Source: CAD feature listing. Evaluate the final solid. Frame: model axes, mm. Coordinates: 2 decimals unless noted, no trailing zeros. Loops run counter-clockwise (first coordinate to the right, second up) from the corner with the lowest first, then second, coordinate; pieces in that order, holes last. Notation, with made-up numbers: M -12,16 L 35,16 A12 cw 35,28 Z; hole C -17.75,87 d9. An arc over 180 degrees is marked long. One line per question, with ' | ' between items. Start each with the question number.
1. Section query C-C, the plane x = -10. Output: boundary loops of the cut face in (y, z), and give its area (3 significant figures).
2. Section query A-A, the plane z = -2.5. Output: boundary loops of the cut face in (x, y).
3. Ray query, probe 1 along X at (y, z) = (-2, -7.5); probe 2 along Z at (x, y) = (-10.75, -2.3); probe 3 along X at (y, z) = (-2.1, -5.25). Return the intervals inside material, ascending.
4. Section query B-B, the plane y = -1.2. Output: boundary loops of the cut face in (x, z), and give its area (3 significant figures).
5. Pin query (flat end, axial travel): P1, Ø8, axis at x = 2, z = -15, coming from the +Y side. Return the tip coordinate at first contact, or that it passes through.
```python
from build123d import *

# Parameters (mm, degrees)
CROQUIS1_R        = 1
BRIDA_BASE1_DEPTH = 3


# Sheet-metal steps are written as plain solids
with BuildPart() as part:
    # Croquis1 → Brida base1 (new body)
    with BuildSketch(Plane(origin=(0, 0, 0), x_dir=(1, 0, 0), z_dir=(0, 1, 0))):
        with BuildLine():
            Line((-5.014718626, 0), (5.014718626, 0))
            ThreePointArc((5.014718626, 0), (7.31081922, 0.456722805), (9.257359313, 1.757359313))
            Line((9.257359313, 1.757359313), (10.742640687, 3.242640687))
            ThreePointArc((10.742640687, 3.242640687), (12.043277195, 5.18918078), (12.5, 7.485281374))
            Line((12.5, 7.485281374), (12.5, 25))
            Line((12.5, 25), (-12.5, 25))
            Line((-12.5, 25), (-12.5, 7.485281374))
            ThreePointArc((-12.5, 7.485281374), (-12.043277195, 5.18918078), (-10.742640687, 3.242640687))
            Line((-10.742640687, 3.242640687), (-9.257359313, 1.757359313))
            ThreePointArc((-9.257359313, 1.757359313), (-7.31081922, 0.456722805), (-5.014718626, 0))
        make_face()
        with Locations(Location((-10, 7.5, 0), (0, 0, 270))):
            Circle(CROQUIS1_R, mode=Mode.SUBTRACT)
        with Locations(Location((-5, 2.5, 0), (0, 0, 270))):
            Circle(CROQUIS1_R, mode=Mode.SUBTRACT)
        with Locations(Location((10, 7.5, 0), (0, 0, 270))):
            Circle(CROQUIS1_R, mode=Mode.SUBTRACT)
        with Locations(Location((5, 2.5, 0), (0, 0, 270))):
            Circle(CROQUIS1_R, mode=Mode.SUBTRACT)
    extrude(amount=-BRIDA_BASE1_DEPTH)


solid = part.part
```
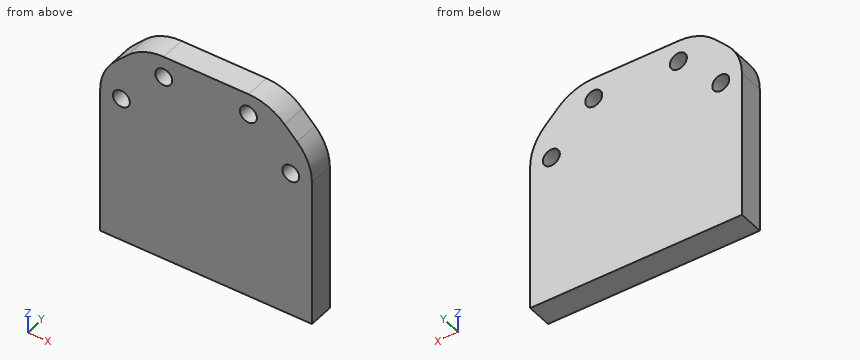
Taken from the geometry:
1) outline: M -3,-25 L 0,-25 L 0,-8.5 L -3,-8.5 Z; M -3,-6.5 L 0,-6.5 L 0,-2.5 L -3,-2.5 Z | area: 61.5 mm^2
2) outline: M -10,-3 L -6,-3 L -6,0 L -10,0 Z; M -4,-3 L 4,-3 L 4,0 L -4,0 Z; M 6,-3 L 10,-3 L 10,0 L 6,0 Z
3) probe 1: -12.5 to -11, -9 to 9, 11 to 12.5 | probe 2: -25 to -8.16, -6.84 to -3.25 | probe 3: -12.07 to 12.07
4) outline: M -12.5,-25 L 12.5,-25 L 12.5,-7.49 A6 ccw 10.74,-3.24 L 9.26,-1.76 A6 ccw 5.01,0 L -5.01,0 A6 ccw -9.26,-1.76 L -10.74,-3.24 A6 ccw -12.5,-7.49 Z; hole C -10,-7.5 d2; hole C -5,-2.5 d2; hole C 5,-2.5 d2; hole C 10,-7.5 d2 | area: 584 mm^2
5) P1: y = 0
